The drawing under review shows one solid part. Ordinate dimensions are in mm from its lowest x, y, z. Coordinates: 2 decimals unless noted, no trailing zeros. Write each loop counter-clockwise with the first axis right and the second up, starting at its lowest first coordinate (ties: lowest second). Pieces come first, ordered by that corner, then holes.
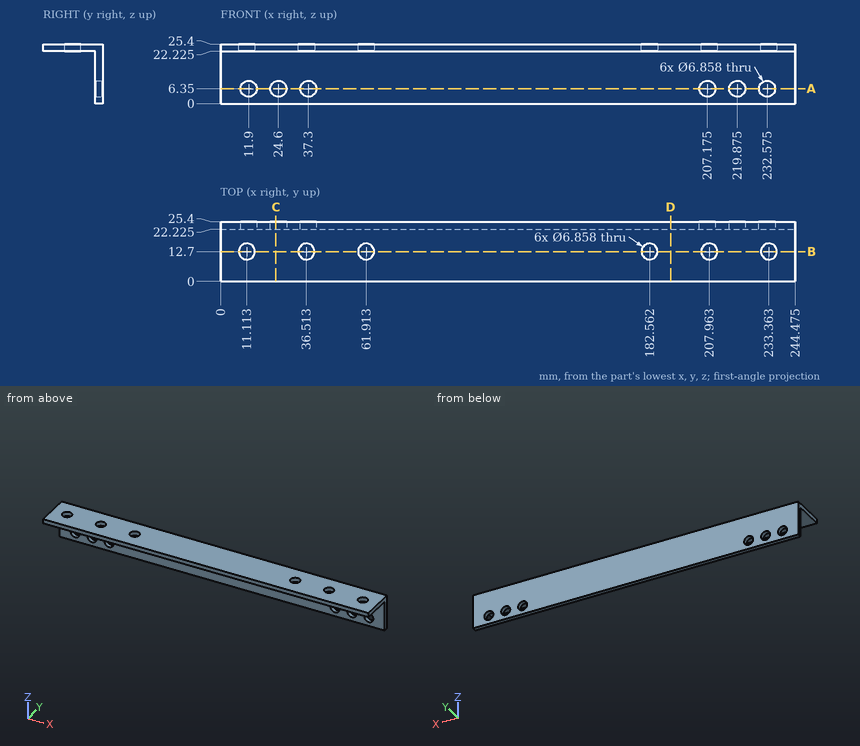
Q1. Add section D-D (x = 191.5). State the section outline as (y, z) points (1 decimal), then the cut area to 3 significant figures.
Ans:
outline: (0, 22.2) - (22.2, 22.2) - (22.2, 0) - (25.4, 0) - (25.4, 25.4) - (0, 25.4) - close
area: 151 mm2
Q2. Add section B-B (y = 12.7). State the section outline as (x, z) points (1 decimal).
Ans:
outline: (0, 22.2) - (7.7, 22.2) - (7.7, 25.4) - (0, 25.4) - close; (14.5, 22.2) - (33.1, 22.2) - (33.1, 25.4) - (14.5, 25.4) - close; (39.9, 22.2) - (58.5, 22.2) - (58.5, 25.4) - (39.9, 25.4) - close; (65.3, 22.2) - (179.1, 22.2) - (179.1, 25.4) - (65.3, 25.4) - close; (186, 22.2) - (204.5, 22.2) - (204.5, 25.4) - (186, 25.4) - close; (211.4, 22.2) - (229.9, 22.2) - (229.9, 25.4) - (211.4, 25.4) - close; (236.8, 22.2) - (244.5, 22.2) - (244.5, 25.4) - (236.8, 25.4) - close
Q3. Add section C-C (x = 23.5). State the section outline as (y, z) points (1 decimal).
Ans:
outline: (0, 22.2) - (22.2, 22.2) - (22.2, 9.6) - (25.4, 9.6) - (25.4, 25.4) - (0, 25.4) - close; (22.2, 0) - (25.4, 0) - (25.4, 3.1) - (22.2, 3.1) - close
Q4. Add section A-A (z = 6.35). State the section outline as (x, y) points (1 decimal).
Ans:
outline: (0, 22.2) - (8.5, 22.2) - (8.5, 25.4) - (0, 25.4) - close; (15.3, 22.2) - (21.2, 22.2) - (21.2, 25.4) - (15.3, 25.4) - close; (28, 22.2) - (33.9, 22.2) - (33.9, 25.4) - (28, 25.4) - close; (40.7, 22.2) - (203.7, 22.2) - (203.7, 25.4) - (40.7, 25.4) - close; (210.6, 22.2) - (216.4, 22.2) - (216.4, 25.4) - (210.6, 25.4) - close; (223.3, 22.2) - (229.1, 22.2) - (229.1, 25.4) - (223.3, 25.4) - close; (236, 22.2) - (244.5, 22.2) - (244.5, 25.4) - (236, 25.4) - close
Q5. For probe 1 along Z at (x, y) = (200, 20.25) (1 decimal), list the stretches that pass through material, from the lowest coordinate up.
Ans:
probe 1: z = 22.2 to 25.4
Q6. Clearance check with flat-ended pins moving along their axes: pin 1 Ø5 at (x, z) = (185.5, 7) entering from -Y (1 decimal); pin 2 Ø9 at (x, y) = (233.36, 12.7) entering from -Z (1 decimal); pin 3 Ø3 at (y, z) = (19.5, 15.5) entering from -X. State where each tip first meets the part, or that it passes through.
Ans:
pin 1: stops at y = 22.2
pin 2: stops at z = 22.2
pin 3: passes through
